Check sheet for the modelled part. Datum: model origin and axes. Units: mm. A direction names the side the tool comes from. Coordinates: 2 decimals unless noted, no trailing zeros. Loops run counter-clockwise (first coordinate to the right, second up) from the corner with the lowest first, then second, coordinate; pieces in that order, holes last. Notation, with made-up numbers: M -28.5,-32 L -2.5,-32 A24 cw -2.5,-7 Z; hole C -17,-23.5 d4. An arc over 180 degrees is marked long. Use CSV: the item, a comma, the result in double quotes. Start each with the question number.
(1) Section check B-B on x = -1.25. Record the cut outline in (y, z), and give its area (3 significant figures).
(2) Section check D-D on z = 1.75. Record the cut outline in (x, y), and give its area (3 significant figures).
(3) Set-up check for faces 1 (the flat face through (12, 0, 6)), 2 (the flat face through (17, 7, -8)), 3 (the flat face through (10, 1, -2.5)), 4 (the flat face through (12, 0, -6)): record each of +Z, -Z, +X, -X, +Y, -Y from which the full face is reachable in a straight line by a thin tool's end or side.
(4) Scan lines: line 1 (Z direction, x = 0.25, y = 0.75); line 2 (Z direction, x = 7, y = 0.5); line 3 (X direction, y = 8.75, z = -2.5). Record each from-to range of solid material in increasing order.
(5) Section check A-A on y = 1.75. Record the cut outline in (x, z), and give its area (3 significant figures).
(6) Draft check along Z on faces 5 (the flat face through (18, 7, 7)), 6 (the flat face through (0, -5, -6)), 7 (the flat face through (-7, 5, 0)). Enter one of: pulls with the +Z half, pulls with the -Z half, needs draft (parallel to the pull), parting line crosses it, or undercut.
(7) Section check C-C on y = 7. Record the cut outline in (x, z).
(8) Go/stop test with flat-tipped pins: pin 1 Ø10 at (x, z) = (15.5, -4) entering from -Y; pin 2 Ø4.5 at (x, y) = (-6, 2.5) entering from -Z; pin 3 Ø2 at (x, z) = (5, 1) entering from -Y. Record where each tip stops, or that it passes through.
from build123d import *

# Parameters (mm, degrees)
F1_DEPTH = 5
F2_DEPTH = 15
F3_DEPTH = 5


with BuildPart() as f1:
    # F0 (on Front) → F1 (new body)
    with BuildSketch(Plane.XZ):
        with BuildLine():
            ThreePointArc((-4.3301270189, 2.5), (0, 5), (4.3301270189, 2.5))
            Line((4.3301270189, 2.5), (9.6824583655, 2.5))
            ThreePointArc((9.6824583655, 2.5), (6.123724357, 7.9056941504), (0, 10))
            ThreePointArc((0, 10), (-6.123724357, 7.9056941504), (-9.6824583655, 2.5))
            Line((-9.6824583655, 2.5), (-4.3301270189, 2.5))
        make_face()
    extrude(amount=F1_DEPTH)



with BuildPart() as f1b:
    # F0 (on Front) → F1, piece 2 (new body)
    with BuildSketch(Plane.XZ):
        with BuildLine():
            Line((9.6824583655, -2.5), (4.3301270189, -2.5))
            ThreePointArc((4.3301270189, -2.5), (0, -5), (-4.3301270189, -2.5))
            Line((-4.3301270189, -2.5), (-9.6824583655, -2.5))
            ThreePointArc((-9.6824583655, -2.5), (-6.123724357, -7.9056941504), (0, -10))
            ThreePointArc((0, -10), (6.123724357, -7.9056941504), (9.6824583655, -2.5))
        make_face()
    extrude(amount=F1_DEPTH)


with BuildPart() as f1_1:
    add(f1.part)

    add(f1b.part)  # F2 merges F1b
    # F0 (on Front) → F2 (join)
    with BuildSketch(Plane.XZ):
        with BuildLine():
            ThreePointArc((0, 10), (6.123724357, 7.9056941504), (9.6824583655, 2.5))
            Line((9.6824583655, 2.5), (20, 2.5))
            Line((20, 2.5), (20, 5))
            Line((20, 5), (15, 10))
            Line((15, 10), (0, 10))
        make_face()
        with BuildLine():
            ThreePointArc((4.3301270189, 2.5), (4.8296291314, 1.2940952255), (5, 0))
            ThreePointArc((5, 0), (4.8296291314, -1.2940952255), (4.3301270189, -2.5))
            Line((4.3301270189, -2.5), (9.6824583655, -2.5))
            Line((9.6824583655, -2.5), (20, -2.5))
            Line((20, -2.5), (20, 2.5))
            Line((20, 2.5), (9.6824583655, 2.5))
            Line((9.6824583655, 2.5), (4.3301270189, 2.5))
        make_face()
        with BuildLine():
            ThreePointArc((-4.3301270189, -2.5), (-5, 0), (-4.3301270189, 2.5))
            Line((-4.3301270189, 2.5), (-9.6824583655, 2.5))
            ThreePointArc((-9.6824583655, 2.5), (-10, 0), (-9.6824583655, -2.5))
            Line((-9.6824583655, -2.5), (-4.3301270189, -2.5))
        make_face()
        with BuildLine():
            Line((20, -2.5), (9.6824583655, -2.5))
            ThreePointArc((9.6824583655, -2.5), (6.123724357, -7.9056941504), (0, -10))
            Line((0, -10), (15, -10))
            Line((15, -10), (20, -5))
            Line((20, -5), (20, -2.5))
        make_face()
        with BuildLine():
            ThreePointArc((-4.3301270189, 2.5), (0, 5), (4.3301270189, 2.5))
            Line((4.3301270189, 2.5), (9.6824583655, 2.5))
            ThreePointArc((9.6824583655, 2.5), (6.123724357, 7.9056941504), (0, 10))
            ThreePointArc((0, 10), (-6.123724357, 7.9056941504), (-9.6824583655, 2.5))
            Line((-9.6824583655, 2.5), (-4.3301270189, 2.5))
        make_face()
        with BuildLine():
            Line((9.6824583655, -2.5), (4.3301270189, -2.5))
            ThreePointArc((4.3301270189, -2.5), (0, -5), (-4.3301270189, -2.5))
            Line((-4.3301270189, -2.5), (-9.6824583655, -2.5))
            ThreePointArc((-9.6824583655, -2.5), (-6.123724357, -7.9056941504), (0, -10))
            ThreePointArc((0, -10), (6.123724357, -7.9056941504), (9.6824583655, -2.5))
        make_face()
    extrude(amount=-F2_DEPTH)

    # F0 (on Front) → F3 (cut)
    with BuildSketch(Plane.XZ):
        with BuildLine():
            ThreePointArc((4.3301270189, 2.5), (4.8296291314, 1.2940952255), (5, 0))
            ThreePointArc((5, 0), (4.8296291314, -1.2940952255), (4.3301270189, -2.5))
            Line((4.3301270189, -2.5), (9.6824583655, -2.5))
            Line((9.6824583655, -2.5), (20, -2.5))
            Line((20, -2.5), (20, 2.5))
            Line((20, 2.5), (9.6824583655, 2.5))
            Line((9.6824583655, 2.5), (4.3301270189, 2.5))
        make_face()
        with BuildLine():
            ThreePointArc((-4.3301270189, -2.5), (-5, 0), (-4.3301270189, 2.5))
            Line((-4.3301270189, 2.5), (-9.6824583655, 2.5))
            ThreePointArc((-9.6824583655, 2.5), (-10, 0), (-9.6824583655, -2.5))
            Line((-9.6824583655, -2.5), (-4.3301270189, -2.5))
        make_face()
    extrude(amount=-F3_DEPTH, mode=Mode.SUBTRACT)


solid = f1_1.part
Outcome:
1,outline,"M -5,-9.92 L 15,-9.92 L 15,-4.84 L -5,-4.84 Z; M -5,4.84 L 15,4.84 L 15,9.92 L -5,9.92 Z"
1,area,"203 mm²"
2,outline,"M -9.85,5 L -4.68,5 L -4.68,15 L -9.85,15 Z; M 4.68,5 L 20,5 L 20,15 L 4.68,15 Z"
2,area,"205 mm²"
3,face 1,"+Z, +X, -Y"
3,face 2,"-Z, +X, +Y, -Y"
3,face 3,"+X, -X, -Y"
3,face 4,"-Z, +X, -Y"
4,line 1,"z = -10 to -4.99, 4.99 to 10"
4,line 2,"z = -10 to -2.5, 2.5 to 10"
4,line 3,"x = -9.68 to -4.33, 4.33 to 20"
5,outline,"M -9.68,-2.5 A10 ccw 0,-10 L 15,-10 L 20,-5 L 20,-2.5 L 4.33,-2.5 A5 cw -4.33,-2.5 Z; M -9.68,2.5 L -4.33,2.5 A5 cw 4.33,2.5 L 20,2.5 L 20,5 L 15,10 L 0,10 A10 ccw Z"
5,area,"352 mm²"
6,face 5,"pulls with the +Z half"
6,face 6,"needs draft"
6,face 7,"undercut"
7,outline,"M 0,-10 L 15,-10 L 20,-5 L 20,5 L 15,10 L 0,10 A10 ccw Z; hole C 0,0 d10"
8,pin 1,"stops at y = 0"
8,pin 2,"stops at z = -9.27"
8,pin 3,"stops at y = 5"
